Autodesk Inventor part; units mm, degrees
ref_plane "YZ Plane" through (0, 0, 0) normal (1, 0, 0) x (0, 1, 0)
ref_plane "XZ Plane" through (0, 0, 0) normal (0, 1, 0) x (-1, 0, 0)
ref_plane "XY Plane" through (0, 0, 0) normal (0, 0, 1) x (1, 0, 0)
sketch "草图2" plane through (0, 0, 0) normal (0, 1, 0) x (-1, 0, 0)
  line L0 (-20, 30) -> (20, 30)
  line L1 (20, 30) -> (20, -30)
  line L2 (20, -30) -> (-20, -30)
  line L3 (-20, -30) -> (-20, 30)
  line L4 (-20, 30) -> (20, -30) construction
  line L5 (20, 30) -> (-20, -30) construction
  point P0 (0, 0)
  dimension "d15" = 40
  dimension "d16" = 60
extrude "拉伸2" add sketch "草图2" along normal blind 30
shell "抽壳1" thickness 2 removed faces 1 at (-6.6667, 0, -10)
sketch "草图3" plane through (-20, 0, 30) normal (0, 0, 1) x (1, 0, 0)
  line L0 (40, 0) -> (0, 0) construction
  line L1 (40, 0) -> (40, 30) construction
  line L2 (0, 30) -> (40, 30) construction
  line L3 (0, 0) -> (0, 30) construction
  line L4 (0, 0) -> (0, 30) construction
  line L5 (40, 0) -> (40, 30) construction
  line L6 (40, 0) -> (0, 0) construction
  line L7 (3, 6.7398) -> (1, 6.7398)
  line L8 (1, 6.7398) -> (1, 0.7398)
  line L9 (0, 1.7398) -> (40, 1.7398) construction
  line L10 (3, 6.7398) -> (3, 2.7398)
  line L11 (40, 30) -> (0, 30) construction
  line L12 (20, 30) -> (20, 0) construction
  line L13 (38, 0) -> (2, 0)
  line L14 (3, 2.7398) -> (20, 2.7398)
  line L15 (1, 0.7398) -> (20, 0.7398)
  line L16 (37, 6.7398) -> (39, 6.7398)
  line L17 (39, 6.7398) -> (39, 0.7398)
  line L18 (37, 6.7398) -> (37, 2.7398)
  line L19 (37, 2.7398) -> (20, 2.7398)
  line L20 (39, 0.7398) -> (20, 0.7398)
  point P0 (20, 0)
  dimension "d29" = 2
  dimension "d44" = 5
  dimension "d45" = 2
  dimension "d46" = 6
  dimension "d47" = 40
extrude "拉伸3" cut sketch "草图3" against normal blind 58
sketch "草图5" plane through (20, 0, 30) normal (1, 0, 0) x (0, 0, -1)
  line L0 (0, 6.7398) -> (58, 6.7398) construction
  line L1 (0, 0.7398) -> (58, 0.7398) construction
  line L2 (0, 6.7398) -> (2, 6.7398) construction
  line L3 (0, 2.7398) -> (2, 2.7398) construction
  line L4 (0, 2.7398) -> (58, 2.7398) construction
  line L5 (58, 6.7398) -> (2, 6.7398) construction
  line L6 (58, 6.7398) -> (58, 0.7398) construction
  line L7 (0, 0) -> (0, 30) construction
  line L8 (0, 4.7398) -> (58, 4.7398) construction
  circle A0 centre (4, 4.7398) radius 1.5
  line L9 (2, 0.7398) -> (2, 6.7398) construction
  circle A1 centre (56, 4.7398) radius 1.5
  point P0 (30, 0)
  dimension "d48" = 4
  dimension "d49" = 3
  dimension "d51" = 2
  dimension "d52" = 2
  dimension "d53" = 3
  dimension "d54" = 2
extrude "拉伸4" cut sketch "草图5" against normal blind 2
mirror "镜像1" about plane through (0, 0, 0) normal (1, 0, 0) of "拉伸4"
sketch "草图7" plane through (-18, 28, 28) normal (0, -1, 0) x (1, 0, 0)
  line L0 (0, 0) -> (36, 0) construction
  line L1 (0, -56) -> (0, 0) construction
  line L2 (36, -56) -> (0, -56) construction
  line L3 (36, 0) -> (36, -56) construction
  line L4 (0.5, -55.5) -> (18.5, -55.5) construction
  line L5 (18.5, -55.5) -> (18.5, -10.5) construction
  line L6 (18.5, -10.5) -> (0.5, -10.5) construction
  line L7 (0.5, -10.5) -> (0.5, -55.5) construction
  circle A0 centre (1.5, -54.5) radius 0.9
  line L8 (3, -56) -> (0, -56)
  line L9 (0, -56) -> (0, -53)
  line L10 (0, -53) -> (3, -53)
  line L11 (3, -53) -> (3, -56)
  line L12 (3, -56) -> (0, -53) construction
  line L13 (0, -56) -> (3, -53) construction
  line L14 (0.5, -55.5) -> (18.5, -10.5) construction
  line L15 (0.5, -10.5) -> (18.5, -55.5) construction
  line L16 (3, -13) -> (0, -13)
  line L17 (0, -13) -> (0, -10)
  line L18 (0, -10) -> (3, -10)
  line L19 (3, -10) -> (3, -13)
  circle A1 centre (1.5, -11.5) radius 0.9
  line L20 (19, -56) -> (16, -56)
  line L21 (16, -56) -> (16, -53)
  line L22 (16, -53) -> (19, -53)
  line L23 (19, -53) -> (19, -56)
  circle A2 centre (17.5, -54.5) radius 0.9
  line L24 (19, -13) -> (16, -13)
  line L25 (16, -13) -> (16, -10)
  line L26 (16, -10) -> (19, -10)
  line L27 (19, -10) -> (19, -13)
  circle A3 centre (17.5, -11.5) radius 0.9
  point P0 (9.5, -33)
  dimension "d70" = 18
  dimension "d71" = 45
  dimension "d79" = 1.8
  dimension "d80" = 1
  dimension "d81" = 1
  dimension "d82" = 3
  dimension "d83" = 3
  dimension "d91" = 43
  dimension "d94" = 16
  dimension "d97" = 1
  dimension "d98" = 1
sketch "草图9" plane through (20, 0, -30) normal (0, 0, -1) x (-1, 0, 0)
  line L0 (37.5, 28) -> (19.5, 28) construction
  line L1 (32, 24.8) -> (25, 24.8)
  line L2 (25, 24.8) -> (25, 28)
  line L3 (25, 28) -> (32, 28)
  line L4 (32, 28) -> (32, 24.8)
  line L5 (32, 24.8) -> (25, 28) construction
  line L6 (25, 24.8) -> (32, 28) construction
  point P0 (20, 0)
  point P1 (28.5, 26.4)
  dimension "d99" = 18
  dimension "d100" = 7
  dimension "d101" = 3.2
  dimension "d102" = 1.6
  dimension "d103" = 9
extrude "拉伸5" add sketch "草图7" along normal blind 3.2
extrude "拉伸6" cut sketch "草图9" against normal blind 2
sketch "草图10" plane through (20, 0, -30) normal (0, 0, -1) x (-1, 0, 0)
  line L0 (32, 28) -> (32, 24.8) construction
  line L1 (32, 24.8) -> (25, 24.8) construction
  line L2 (25, 24.8) -> (25, 28) construction
  line L3 (25, 28) -> (32, 28) construction
  line L4 (40, 0) -> (0, 0) construction
  line L5 (40, 0) -> (40, 30) construction
  line L6 (0, 30) -> (40, 30) construction
  line L7 (0, 0) -> (0, 30) construction
  line L8 (25, 28) -> (25, 24.8) construction
  line L9 (25, 24.8) -> (32, 24.8) construction
  line L10 (32, 24.8) -> (32, 28) construction
  line L11 (32, 28) -> (35, 28) construction
  line L12 (35, 28) -> (35, 24.8) construction
  line L13 (35, 24.8) -> (38, 24.8) construction
  line L14 (38, 6.7398) -> (38, 24.8) construction
  line L15 (39, 6.7398) -> (38, 6.7398) construction
  line L16 (39, 0.7398) -> (39, 6.7398) construction
  line L17 (38, 0.7398) -> (39, 0.7398) construction
  line L18 (38, 0) -> (38, 0.7398) construction
  line L19 (2, 0) -> (38, 0) construction
  line L20 (2, 0) -> (2, 0.7398) construction
  line L21 (1, 0.7398) -> (2, 0.7398) construction
  line L22 (1, 6.7398) -> (1, 0.7398) construction
  line L23 (2, 6.7398) -> (1, 6.7398) construction
  line L24 (2, 6.7398) -> (2, 28) construction
  line L25 (2, 28) -> (19, 28) construction
  line L26 (19, 28) -> (19, 24.8) construction
  line L27 (19, 24.8) -> (22, 24.8) construction
  line L28 (22, 24.8) -> (22, 28) construction
  line L29 (22, 28) -> (25, 28) construction
  circle A0 centre (10.5, 11.2398) radius 7.5
  line L30 (37, 2.7398) -> (3, 2.7398) construction
  line L31 (38, 28) -> (2, 28) construction
  line L32 (10.5, 28) -> (10.5, 0) construction
  line L33 (2, 0) -> (38, 0) construction
  line L34 (5.25, 21.5) -> (15.75, 21.5)
  line L35 (15.75, 21.5) -> (15.75, 26)
  line L36 (15.75, 26) -> (5.25, 26)
  line L37 (5.25, 26) -> (5.25, 21.5)
  line L38 (5.25, 21.5) -> (15.75, 26) construction
  line L39 (15.75, 21.5) -> (5.25, 26) construction
  line L40 (28.5, 24.8) -> (28.5, 2.7398) construction
  line L41 (26.25, 3.9898) -> (30.75, 3.9898)
  line L42 (30.75, 3.9898) -> (30.75, 5.4898)
  line L43 (30.75, 5.4898) -> (26.25, 5.4898)
  line L44 (26.25, 5.4898) -> (26.25, 3.9898)
  line L45 (26.25, 3.9898) -> (30.75, 5.4898) construction
  line L46 (30.75, 3.9898) -> (26.25, 5.4898) construction
  point P0 (20, 0)
  point P1 (10.5, 23.75)
  point P2 (28.5, 4.7398)
  dimension "d108" = 15
  dimension "d111" = 8.5
  dimension "d112" = 17
  dimension "d113" = 10.5
  dimension "d114" = 4.5
  dimension "d115" = 2
  dimension "d116" = 4.5
  dimension "d117" = 1.5
  dimension "d118" = 2
extrude "拉伸7" cut sketch "草图10" against normal blind 2
properties part number "Case"
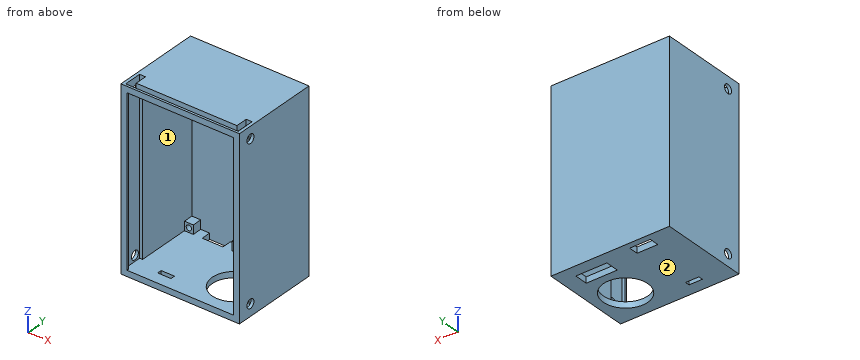
Check sheet for the modelled part. Datum: model origin and axes. Units: mm. Face numbers are marked on the shaded views. A direction names the side the tool comes from. Round coordinates to 2 decimals unless told otherwise and drop trailing zeros. Write each loop counter-clockwise with the first axis right and the second up, starting at its lowest first coordinate (ties: lowest second). Pieces come first, ordered by that corner, then holes. Notation, with made-up numbers: (79.5, 87) - (136.5, 87) arc R23 ccw to (136.5, 121) - close; hole circle Ø5 at (-37, -28.75). An arc over 180 degrees is marked (long way). Return JSON: item names as keys, results as strings.
Q1. Cross-section at D-D (y = 23.5). Record the boundary of the cut face in (x, z).
Returned:
{"outline": "(-20, -30) - (4.25, -30) - (4.25, -28) - (-18, -28) - (-18, 28) - (18, 28) - (18, -28) - (14.75, -28) - (14.75, -30) - (20, -30) - (20, 30) - (-20, 30) - close"}
Q2. Cross-section at A-A (x = 9.5). Record the boundary of the cut face in (y, z).
Returned:
{"outline": "(0, -30) - (3.74, -30) - (3.74, -28) - (0, -28) - close; (0, 28) - (0.74, 28) - (0.74, 30) - (0, 30) - close; (2.74, 28) - (28, 28) - (28, -28) - (26, -28) - (26, -30) - (30, -30) - (30, 30) - (2.74, 30) - close; (18.74, -30) - (21.5, -30) - (21.5, -28) - (18.74, -28) - close"}
Q3. Scan lines: L1, parallel to Y at x = 9.5, z = -29.6; L2, parallel to X at y = 4, z = -9; L3, parallel to X at y = 25.5, z = -14. Record each from-to range of solid material in increasing order. Write a range as from..to.
Returned:
{"L1": "y = 0..3.74, 18.74..21.5, 26..30", "L2": "x = -20..-19, 19..20", "L3": "x = -20..-18, 18..20"}
Q4. Cross-section at C-C (z = 10.5). Record the boundary of the cut face in (x, y), then the cut area to 3 significant figures.
Returned:
{"outline": "(-20, 0) - (-18, 0) - (-18, 0.74) - (-19, 0.74) - (-19, 6.74) - (-18, 6.74) - (-18, 28) - (18, 28) - (18, 6.74) - (19, 6.74) - (19, 0.74) - (18, 0.74) - (18, 0) - (20, 0) - (20, 30) - (-20, 30) - close", "area": "180 mm²"}
Q5. Depth check by flat-ended pin: P1, Ø0.9, axis at x = -1, z = 16.5, coming from the -Y side; P2, Ø6, axis at x = 0.5, z = -2, coming from the -Y side. Enter the tip coordinate at first touch or a pass-through.
Returned:
{"P1": "stops at y = 24.8", "P2": "stops at y = 28"}
Q6. Access from +Z, -Z, +X, -X, +Y, -Y to the whole of each face (thin tool, end or side, straight path). Record for the marked faces 1 and 2.
Returned:
{"face 1": "-Y", "face 2": "-Z, +X, -X, +Y, -Y"}
Q7. Cross-section at B-B (x = -0.5). Record the boundary of the cut face in (y, z), then the cut area to 3 significant figures.
Returned:
{"outline": "(0, -30) - (30, -30) - (30, 30) - (2.74, 30) - (2.74, 28) - (28, 28) - (28, 18) - (24.8, 18) - (24.8, 17.4) - (28, 17.4) - (28, 15.6) - (24.8, 15.6) - (24.8, 15) - (28, 15) - (28, -25) - (24.8, -25) - (24.8, -25.6) - (28, -25.6) - (28, -27.4) - (24.8, -27.4) - (24.8, -28) - (0, -28) - close; (0, 28) - (0.74, 28) - (0.74, 30) - (0, 30) - close", "area": "236 mm²"}
